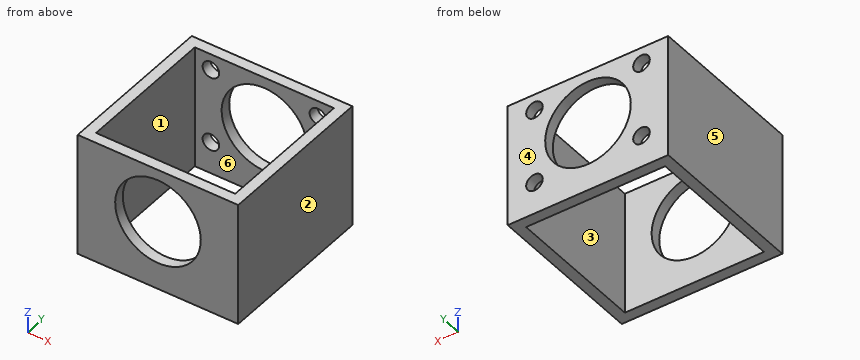
```python
from build123d import *

# Parameters (mm, degrees)
SKETCH1_W               = 30
SKETCH1_H               = 30
SKETCH1_W_2             = 26
SKETCH1_H_2             = 26
BOSS_EXTRUDE1_DEPTH     = 23
CUT_EXTRUDE1_DEPTH      = 30
CUT_EXTRUDE1_DEPTH_BACK = 3
SKETCH2_R               = 8
SKETCH4_R               = 1.55
CUT_EXTRUDE2_DEPTH      = 3


with BuildPart() as part:
    # Sketch1 → Boss-Extrude1 (new body)
    with BuildSketch(Plane.XY):
        Rectangle(SKETCH1_W, SKETCH1_H)
        Rectangle(SKETCH1_W_2, SKETCH1_H_2, mode=Mode.SUBTRACT)
    extrude(amount=BOSS_EXTRUDE1_DEPTH)

    # Sketch2 → Cut-Extrude1 (cut, two sides: drawn at the far end of the back side and taken through both)
    with BuildSketch(Plane(origin=(0, -13, 0), x_dir=(1, 0, 0), z_dir=(0, 1, 0)).offset(-CUT_EXTRUDE1_DEPTH_BACK)):
        with Locations(Location((0, -13, 0), (0, 0, 270))):
            Circle(SKETCH2_R)
    extrude(amount=CUT_EXTRUDE1_DEPTH + CUT_EXTRUDE1_DEPTH_BACK, mode=Mode.SUBTRACT)

    # Sketch4 → Cut-Extrude2 (cut)
    with BuildSketch(Plane(origin=(0, 15, 0), x_dir=(1, 0, 0), z_dir=(0, 1, 0))):
        with Locations(Location((-10, -6, 0), (0, 0, 270))):
            Circle(SKETCH4_R)
        with Locations(Location((10, -6, 0), (0, 0, 270))):
            Circle(SKETCH4_R)
        with Locations(Location((10, -20, 0), (0, 0, 270))):
            Circle(SKETCH4_R)
        with Locations(Location((-10, -20, 0), (0, 0, 270))):
            Circle(SKETCH4_R)
    extrude(amount=-CUT_EXTRUDE2_DEPTH, mode=Mode.SUBTRACT)


solid = part.part
```
Here's how the part is built. I have some questions about the finished solid (model axes, mm). Face numbers are marked on the shaded views. A direction names the side the tool comes from. Coordinates: 2 decimals unless noted, no trailing zeros. Order: outer loops, then holes, each group sorted by start corner. A loop starts at its lowest first (then second) coordinate and runs counter-clockwise, first axis right, second up. Notation, with made-up numbers: M 59,-21.5 L 89,-21.5 A22 ccw 89,-15.5 Z; hole C -17,6.25 d9. An arc over 180 degrees is marked long. Answer as a JSON object with one key per item and string values. Group by question number.
(1) Suppose I cut it at A-A, the plane z = 13. Please give me the cut outline in (x, y), then the cut area to 3 significant figures.
(2) For pin 1 (2.5 mm diameter, centred on x = 10, z = 20, fed in from +Y), with a flat end and sliding along its axis, tell me the tip position at first contact or that it passes through.
(3) If we mould it in two halves opening along X, with no side actions, what happens to the marked faces 3, 4, 5 and 6? For each: released by +X, released by -X, zero draft, split by the parting line, or undercut.
(4) Suppose I cut it at C-C, the plane y = -3. Please give me the cut outline in (x, z).
(5) I need wall thicknesses on probe 1 along X at (y, z) = (-2.5, 13.25); probe 2 along Z at (x, y) = (0, -14.35); probe 3 along X at (y, z) = (-13.5, 13). Which ranges of each line are inside material? Lowest first, please.
(6) Which directions (+Z, -Z, +X, -X, +Y, -Y) give clear straight access to the entire face, cutting with the end or side of a thin tool? Please do the marked faces 1 and 2.
(7) Suppose I cut it at B-B, the plane x = 0. Please give me the cut outline in (y, z).
Values found:
{
 "1": {"outline": "M -15,-15 L -8,-15 L -8,-13 L -13,-13 L -13,13 L -8,13 L -8,15 L -15,15 Z; M 8,-15 L 15,-15 L 15,15 L 8,15 L 8,13 L 13,13 L 13,-13 L 8,-13 Z", "area": "160 mm^2"},
 "2": {"pin 1": "stops at y = -13"},
 "3": {"face 3": "undercut", "face 4": "zero draft", "face 5": "released by -X", "face 6": "undercut"},
 "4": {"outline": "M -15,0 L -13,0 L -13,23 L -15,23 Z; M 13,0 L 15,0 L 15,23 L 13,23 Z"},
 "5": {"probe 1": "x = -15 to -13, 13 to 15", "probe 2": "z = 0 to 5, 21 to 23", "probe 3": "x = -15 to -8, 8 to 15"},
 "6": {"face 1": "+Z, -Z", "face 2": "+Z, -Z, +X, +Y, -Y"},
 "7": {"outline": "M -15,0 L -13,0 L -13,5 L -15,5 Z; M -15,21 L -13,21 L -13,23 L -15,23 Z; M 13,0 L 15,0 L 15,5 L 13,5 Z; M 13,21 L 15,21 L 15,23 L 13,23 Z"}
}
